```python
from build123d import *

# Parameters (mm, degrees)
SKETCH001_R        = 12
SKETCH001_R_2      = 4.5
POCKET_DEPTH       = 210.001
POLARPATTERN_COUNT = 4
POCKET001_DEPTH    = 4
CHAMFER_SIZE       = 0.5


with BuildPart() as part:
    # Sketch → Revolution (revolve)
    with BuildSketch(Plane.XZ):
        Polygon((0, 2), (-5.985281, 2), (-8, 0), (-29.955844, 0), (-32.977922, 3), (-36, 3), (-36, 2.12132), (-33.87868, 0), (-36, -2.12132), (-36, -3), (0, -3), align=None)
    revolve(axis=Axis((0, 0, 0), (0, 0, 1)))

    # Sketch001 → Pocket (cut, through all)
    with BuildSketch(Plane(origin=(0, 0, -3), x_dir=(1, 0, 0), z_dir=(0, 0, -1))):
        with Locations((0, 20)):
            Circle(SKETCH001_R)
        with Locations((18, 18)):
            Circle(SKETCH001_R_2)
    pocket = extrude(amount=-POCKET_DEPTH, mode=Mode.SUBTRACT)

    # PolarPattern: Pocket ×4 about axis
    polarpattern_axis = Axis((0, 0, -3), (0, 0, -1))
    for i in range(1, POLARPATTERN_COUNT):
        add(pocket.rotate(polarpattern_axis, i * 360 / POLARPATTERN_COUNT), mode=Mode.SUBTRACT)

    # Sketch002 → Pocket001 (cut)
    with BuildSketch(Plane(origin=(0, 0, -3), x_dir=(1, 0, 0), z_dir=(0, 0, -1))):
        with BuildLine():
            ThreePointArc((-2, 1.5), (-2.5, 0), (-2, -1.5))
            Line((2, -1.5), (-2, -1.5))
            ThreePointArc((2, -1.5), (2.5, 0), (2, 1.5))
            Line((2, 1.5), (-2, 1.5))
        make_face()
    extrude(amount=-POCKET001_DEPTH, mode=Mode.SUBTRACT)

    # Chamfer
    chamfer_edges = [part.edges().sort_by_distance(p)[0] for p in [
        (0, -1.5, -3),
        (-2.5, 0, -3),
        (0, 1.5, -3),
        (2.5, 0, -3),
    ]]
    chamfer(chamfer_edges, length=CHAMFER_SIZE)


solid = part.part
```
Build history of the part. All positions in model axes, mm. A direction names the side the tool comes from. Give positions to 0.01 mm unless a question says otherwise; leave off trailing zeros.
1) Band-saw the part on A-A on x = -20. State how many separate pieces and enclosed holes the cut face has, then the cut area to 3 significant figures.
Values follow:
separate pieces: 4
enclosed holes: 0
area: 82.2 mm2
2) Drop flat-ended pins along their axis: P1, Ø3, axis at x = -1, z = 0, coming from the -Y side; P2, Ø8.5, axis at x = -9.5, y = -11, coming from the +Z side; P3, Ø1.8, axis at x = 0, z = -1.5, coming from the +Y side. Give the stop position or say it passes through.
Values follow:
P1: stops at y = -35.37
P2: stops at z = 0
P3: stops at y = 36
3) 3-axis set-ups, long thin cutter, end or side, ignore diameter. For faces 1 (the face through (-14, -14, 0)), 2 (the face through (0, -1.5, -1)), 3 (the face through (-32.441, -10.216, -0.133)): which of +Z, -Z, +X, -X, +Y, -Y reach the whole face in a straight line?
Values follow:
face 1: +Z
face 2: -Z
face 3: none
4) Two-plate mould, pull along X, no slides. Class faces 4 (the face through (-2.5, 0, -0.8)), 5 (the face through (4.686, -35.694, 2.555)), 6 (the face through (15.8, 29.2, 3)): released by +X, released by -X, zero draft, split by the parting line, or undercut.
Values follow:
face 4: undercut
face 5: split by the parting line
face 6: zero draft
5) Probe line 1 along Y through (x, z) = (18, -1.25); line 2 along X through (y, z) = (20, -0.15); line 3 along X through (y, z) = (20, -1.3). List the from-to ranges inside material, lowest first.
Values follow:
line 1: y = -30.17 to -22.5, -13.5 to -11.83, 11.83 to 13.5, 22.5 to 30.17
line 2: x = -27.53 to -22.03, -13.97 to -12, 12 to 13.97, 22.03 to 27.53
line 3: x = -28.94 to -22.03, -13.97 to -12, 12 to 13.97, 22.03 to 28.94
